Answer from the drawing. Dimensions are ordinates in mm from the lowest x, y and z of the part. A direction names the side the tool comes from. Coordinates: 2 decimals unless noted, no trailing zeros. Order: outer loops, then holes, each group sorted by start corner. A loop starts at its lowest first (then second) coordinate and runs counter-clockwise, first axis right, second up. Notation, with made-up numbers: (-35.5, 10) - (-28.5, 10) arc R24 cw to (-28.5, 30) - close; hole circle Ø11 at (31.5, 40). An arc over 180 degrees is marked (long way). Use a Markdown table: item, result. Add a question column.
Item 1: The part is cut by section A-A, the plane z = 10.2. Give the vertices of the cut face in (x, y) (3 decimals).
Item 2: The mould has two halves that part along Z. Classify the marked faces 3, 4, 5 and 6: released by +Z, released by -Z, zero draft, split by the parting line, or undercut.
Item 3: A flat-ended cylindrical pin translates along its axis: P1, Ø5.5, axis at y = 10.2, z = 10.2, coming from the +X side (3 decimals). Find the tip coordinate at first contact, or state that the pin passes through.
Item 4: The part is cut by section C-C, the plane x = 7. Give the vertices of the cut face in (y, z), then the cut area to 3 significant figures.
Item 5: Find the intervals of material crossed by line 1 along Y through (x, z) = (11, 10.2); line 2 along Y through (x, z) = (3.75, 10.2) (3 decimals); line 3 along X through (y, z) = (17, 1.75), in increasing order.
Item 6: For the marked faces 1 and 2, determine the directions among +Z, -Z, +X, -X, +Y, -Y from which every point of the face is accessible in a straight line to the end or side of a thin tool.
Item 7: The part is cut by section D-D, the plane y = 14.75. Give the vertices of the cut face in (x, z), then the cut area to 3 significant figures.
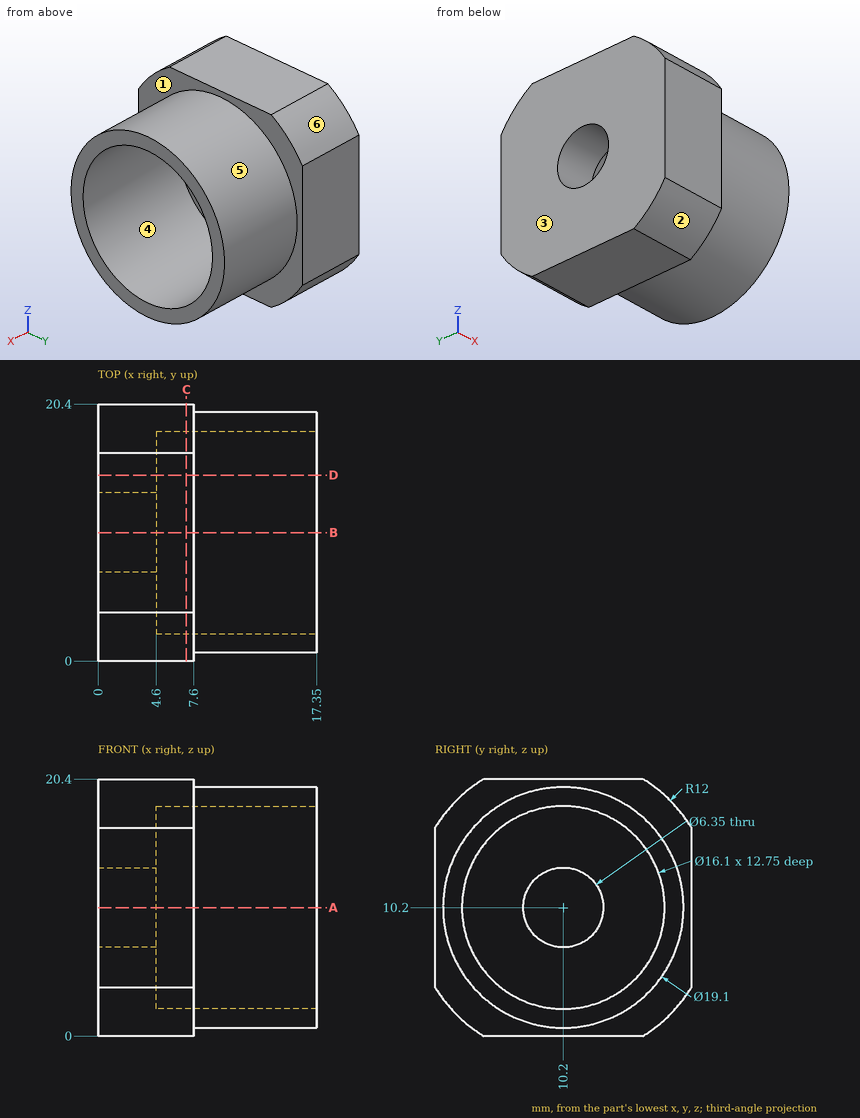
Solution:
| question | item | result |
|---|---|---|
| 1 | outline | (0, 0) - (7.6, 0) - (7.6, 0.65) - (17.35, 0.65) - (17.35, 2.15) - (4.6, 2.15) - (4.6, 7.025) - (0, 7.025) - close; (0, 13.375) - (4.6, 13.375) - (4.6, 18.25) - (17.35, 18.25) - (17.35, 19.75) - (7.6, 19.75) - (7.6, 20.4) - (0, 20.4) - close |
| 2 | face 3 | zero draft |
| 2 | face 4 | undercut |
| 2 | face 5 | split by the parting line |
| 2 | face 6 | released by +Z |
| 3 | P1 | passes through |
| 4 | outline | (0, 3.88) arc R12 ccw to (3.88, 0) - (16.52, 0) arc R12 ccw to (20.4, 3.88) - (20.4, 16.52) arc R12 ccw to (16.52, 20.4) - (3.88, 20.4) arc R12 ccw to (0, 16.52) - close; hole circle Ø16.1 at (10.2, 10.2) |
| 4 | area | 187 mm2 |
| 5 | line 1 | y = 0.65 to 2.15, 18.25 to 19.75 |
| 5 | line 2 | y = 0 to 7.025, 13.375 to 20.4 |
| 5 | line 3 | x = 0 to 7.6 |
| 6 | face 1 | +X |
| 6 | face 2 | -Z, +X, -X, -Y |
| 7 | outline | (0, 0) - (7.6, 0) - (7.6, 1.8) - (17.35, 1.8) - (17.35, 3.56) - (4.6, 3.56) - (4.6, 16.84) - (17.35, 16.84) - (17.35, 18.6) - (7.6, 18.6) - (7.6, 20.4) - (0, 20.4) - close |
| 7 | area | 149 mm2 |
